Geometry check sheet. Reference: the model listing, model coordinates, mm. A direction names the side the tool comes from. Give positions to 0.01 mm unless a question says otherwise; leave off trailing zeros. Write each loop counter-clockwise with the first axis right and the second up, starting at its lowest first coordinate (ties: lowest second). Pieces come first, ordered by that corner, then holes. Notation, with made-up numbers: (67, 43.5) -> (106, 43.5) arc R29 ccw to (106, 78.5) -> close; hole circle Ø4 at (41, 73.5). An arc over 180 degrees is marked (long way). One line per item, written item: value.
from build123d import *

# Parameters (mm, degrees)
SKETCH1_R           = 15
BOSS_EXTRUDE1_DEPTH = 50


with BuildPart() as part:
    # Sketch1 → Boss-Extrude1 (new body)
    with BuildSketch(Plane.XY):
        with BuildLine():
            ThreePointArc((-60, 40), (-30, 70), (0, 40))
            Line((0, 40), (0, 0))
            Line((0, 0), (-150, 0))
            Line((-150, 0), (-150, 20))
            Line((-150, 20), (-115, 20))
            Line((-115, 20), (-115, 15))
            Line((-115, 15), (-90, 15))
            Line((-90, 15), (-90, 20))
            Line((-90, 20), (-60, 20))
            Line((-60, 20), (-60, 40))
        make_face()
        with Locations((-30, 40)):
            Circle(SKETCH1_R, mode=Mode.SUBTRACT)
    extrude(amount=BOSS_EXTRUDE1_DEPTH)


solid = part.part
1) Scan lines: probe 1 along Y at (x, z) = (-30, 23); probe 2 along Y at (x, z) = (-132, 2); probe 3 along X at (y, z) = (30, 15). Record each from-to range of solid material in increasing order.
Verdict:
probe 1: 0 to 25, 55 to 70
probe 2: 0 to 20
probe 3: -60 to -41.18, -18.82 to 0
2) Sectioned sample at A-A on z = 29. Record the cut outline in (x, y), plus the area to 3 significant figures.
Verdict:
outline: (-150, 0) -> (0, 0) -> (0, 40) arc R30 ccw to (-60, 40) -> (-60, 20) -> (-90, 20) -> (-90, 15) -> (-115, 15) -> (-115, 20) -> (-150, 20) -> close; hole circle Ø30 at (-30, 40)
area: 4,780 mm^2
3) Sectioned sample at C-C on y = 27. Record the cut outline in (x, z), plus the area to 3 significant figures.
Verdict:
outline: (-60, 0) -> (-37.48, 0) -> (-37.48, 50) -> (-60, 50) -> close; (-22.52, 0) -> (0, 0) -> (0, 50) -> (-22.52, 50) -> close
area: 2,250 mm^2
4) Tool access check on faces 1 (the flat face through (-90, 17, 25)), 2 (the flat face through (-75, 20, 25)), 3 (the flat face through (-57, 28, 50)). Record the directions out of +Z, -Z, +X, -X, +Y, -Y that give a thin tool (end or side, any length) a straight path to the whole face; none if there is none.
Verdict:
face 1: +Z, -Z, +Y
face 2: +Z, -Z, -X, +Y
face 3: +Z, +X, -X, +Y, -Y
5) Depth check by flat-ended pin: pin 1 Ø10 at (x, z) = (-96.5, 19.5) entering from +Y; pin 2 Ø24 at (x, z) = (-79.5, 19.5) entering from +Y; pin 3 Ø4 at (x, z) = (-46.5, 31) entering from +Y. Enter the tip coordinate at first touch or a pass-through.
Verdict:
pin 1: y = 15
pin 2: y = 20
pin 3: y = 66.26
6) Sectioned sample at D-D on x = -117. Record the cut outline in (y, z), plus the area to 3 significant figures.
Verdict:
outline: (0, 0) -> (20, 0) -> (20, 50) -> (0, 50) -> close
area: 1,000 mm^2
7) Sectioned sample at B-B on x = -30. Record the cut outline in (y, z).
Verdict:
outline: (0, 0) -> (25, 0) -> (25, 50) -> (0, 50) -> close; (55, 0) -> (70, 0) -> (70, 50) -> (55, 50) -> close
